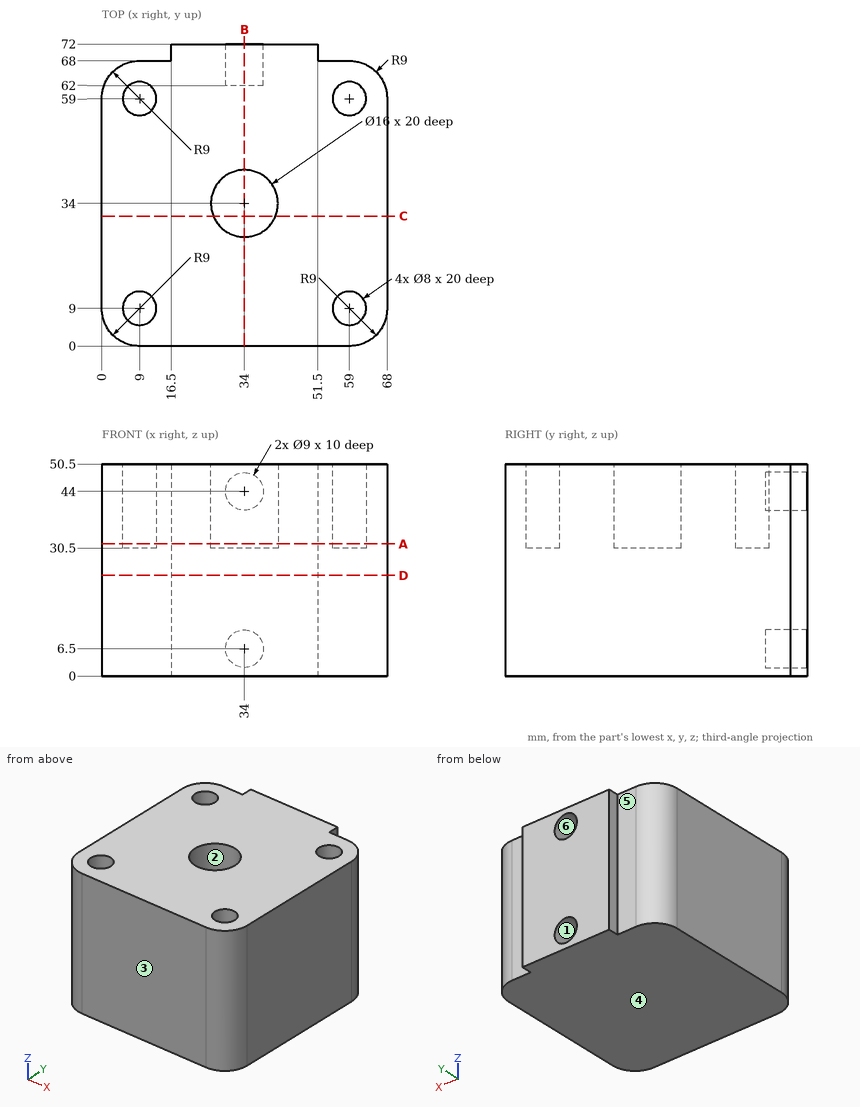
Geometry: see drawing. Coordinates: mm, zero at the bounding-box minimum. A direction names the side the tool comes from. Round coordinates to 2 decimals unless told otherwise and drop trailing zeros. Write each loop counter-clockwise with the first axis right and the second up, starting at its lowest first coordinate (ties: lowest second). Pieces come first, ordered by that corner, then holes. Notation, with made-up numbers: M -10,75.25 L 32,75.25 A35 cw 32,111.25 Z; hole C -1.75,76.25 d7. An arc over 180 degrees is marked long. Answer as a JSON object with one key per item and string values. Group by question number.
(1) Section query C-C on y = 31. Output: boundary loops of the cut face in (x, z).
(2) Section query D-D on z = 24. Output: boundary loops of the cut face in (x, y).
(3) Section query A-A on z = 31.5. Output: boundary loops of the cut face in (x, y), then the cut area to 3 significant figures.
(4) Reachability of the marked faces 4, 5 and 6 from +Z, -Z, +X, -X, +Y, -Y: full face, straight path, thin tool, end or side. Return the list, or none.
(5) Section query B-B on x = 34. Output: boundary loops of the cut face in (y, z), then the cut area to 3 significant figures.
(6) Mould query, pull axis Y, two halves, no side actions, for the marked faces 1, 2 and 3. Classes: +Y half, -Y half, draft (parallel to the pull), parting line (faces both ways), or undercut.
(7) First-contact query: pin 1 (1 mm diameter, centred on x = 59, y = 11, fed in from -Z); pin 2 (2 mm diameter, centred on y = 69.5, z = 36, fed in from -X); pin 3 (6.5 mm diameter, centred on x = 58.5, y = 9, fed in from +Z); pin 4 (2.5 mm diameter, centred on x = 36, z = 44, fed in from +Y). Flat tips, straight axial feed; report the tip coordinate or a pass-through.
(8) Ray query, line 1 (Y direction, x = 59, z = 35.25); line 2 (Y direction, x = 34, z = 38.5); line 3 (X direction, y = 6, z = 35). Return the intervals inside material, ascending. Write a range as [from, to].
Computed values:
{
 "1": {"outline": "M 0,0 L 68,0 L 68,50.5 L 41.42,50.5 L 41.42,30.5 L 26.58,30.5 L 26.58,50.5 L 0,50.5 Z"},
 "2": {"outline": "M 0,9 A9 ccw 9,0 L 59,0 A9 ccw 68,9 L 68,59 A9 ccw 59,68 L 51.5,68 L 51.5,72 L 16.5,72 L 16.5,68 L 9,68 A9 ccw 0,59 Z"},
 "3": {"outline": "M 0,9 A9 ccw 9,0 L 59,0 A9 ccw 68,9 L 68,59 A9 ccw 59,68 L 51.5,68 L 51.5,72 L 16.5,72 L 16.5,68 L 9,68 A9 ccw 0,59 Z; hole C 9,9 d8; hole C 9,59 d8; hole C 34,34 d16; hole C 59,9 d8; hole C 59,59 d8", "area": "4,290 mm^2"},
 "4": {"face 4": "-Z, +X, -X, +Y, -Y", "face 5": "+Z, -Z, -X, +Y", "face 6": "+Y"},
 "5": {"outline": "M 0,0 L 72,0 L 72,2 L 62,2 L 62,11 L 72,11 L 72,39.5 L 62,39.5 L 62,48.5 L 72,48.5 L 72,50.5 L 42,50.5 L 42,30.5 L 26,30.5 L 26,50.5 L 0,50.5 Z", "area": "3,140 mm^2"},
 "6": {"face 1": "draft", "face 2": "undercut", "face 3": "-Y half"},
 "7": {"pin 1": "z = 0", "pin 2": "x = 16.5", "pin 3": "z = 30.5", "pin 4": "y = 62"},
 "8": {"line 1": "[0, 5], [13, 55], [63, 68]", "line 2": "[0, 26], [42, 72]", "line 3": "[0.51, 6.35], [11.65, 56.35], [61.65, 67.49]"}
}
